The drawing under review shows one solid part. Ordinate dimensions are in mm from its lowest x, y, z. Round coordinates to 2 decimals unless told otherwise and drop trailing zeros. Loops run counter-clockwise (first coordinate to the right, second up) from the corner with the lowest first, then second, coordinate; pieces in that order, holes last. Notation, with made-up numbers: (0.5, -17.5) - (6.5, -17.5) arc R17 ccw to (6.5, 14.5) - close; hole circle Ø2 at (40, -13). An arc over 180 degrees is marked (long way). Answer as CSV lines item,"result".
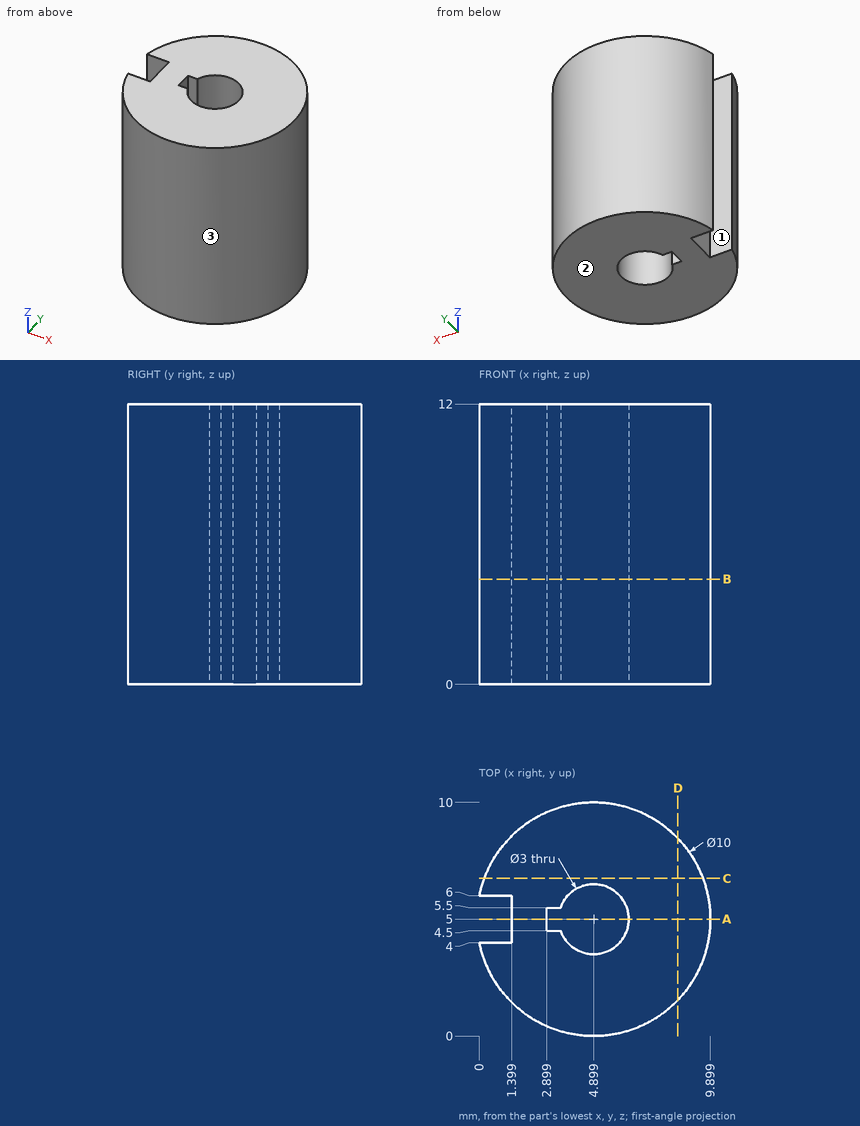
1. Take a section at B-B (z = 4.5). State the section outline as (x, y) points.
Numbers:
outline,"(0, 4) arc R5 ccw (long way) to (0, 6) - (1.4, 6) - (1.4, 4) - close; hole (2.9, 4.5) - (3.48, 4.5) arc R1.5 ccw (long way) to (3.48, 5.5) - (2.9, 5.5) - close"
2. Draft analysis for pull direction Y (two halves, no side actions). For the marked faces 1, 2 and 3, state which applies: +Y half, -Y half, draft (parallel to the pull), parting line (faces both ways), or undercut.
Numbers:
face 1,"undercut"
face 2,"draft"
face 3,"parting line"
3. Wall thickness on probe 1 along X at (y, z) = (5, 9.25); probe 2 along Y at (x, z) = (6, 2.5); probe 3 along Y at (x, z) = (5.75, 11.25): over which ranges is each line inside the solid? List them lowest first.
Numbers:
probe 1,"x = 1.4 to 2.9, 6.4 to 9.9"
probe 2,"y = 0.12 to 3.98, 6.02 to 9.88"
probe 3,"y = 0.07 to 3.76, 6.24 to 9.93"
4. Take a section at D-D (x = 8.5). State the section outline as (y, z) points.
Numbers:
outline,"(1.53, 0) - (8.47, 0) - (8.47, 12) - (1.53, 12) - close"
5. Clearance check with flat-ended pins moving along their axes: pin 1 (1.1 mm diameter, centred on x = 1, z = 6, fed in from +Y); pin 2 (0.6 mm diameter, centred on x = 3, z = 3.5, fed in from -Y); pin 3 (0.7 mm diameter, centred on x = 1, z = 6.5, fed in from -Y); pin 4 (4 mm diameter, centred on x = 4.5, z = 7.5, fed in from +Y). State where each tip first meets the part, or that it passes through.
Numbers:
pin 1,"stops at y = 8.71"
pin 2,"stops at y = 0.26"
pin 3,"stops at y = 1.48"
pin 4,"stops at y = 10"
6. Take a section at A-A (y = 5). State the section outline as (x, z) points, plus the area to 3 significant figures.
Numbers:
outline,"(1.4, 0) - (2.9, 0) - (2.9, 12) - (1.4, 12) - close; (6.4, 0) - (9.9, 0) - (9.9, 12) - (6.4, 12) - close"
area,"60.0 mm²"
7. Take a section at C-C (y = 6.75). State the section outline as (x, z) points.
Numbers:
outline,"(0.22, 0) - (9.58, 0) - (9.58, 12) - (0.22, 12) - close"
